Verification items for the finished model (mm, model axes). Face numbers are marked on the shaded views. A direction names the side the tool comes from. Give positions to 0.01 mm unless a question says otherwise; leave off trailing zeros. Answer as a JSON object with one key per item and string values. Group by question number.
(1) Mould release check, pull along Y, two halves, no side actions. Record for the marked faces 1 and 2: +Y half, -Y half, draft (parallel to the pull), parting line (faces both ways), or undercut.
(2) Section check A-A (z = 7.25). Count the separate pieces of the cut face and the enclosed holes in it, then the cut area to 3 significant figures.
(3) Thickness scan on line 1 (Y direction, x = 14, z = 4.5); line 2 (Y direction, x = -0.5, z = 9.5); line 3 (Z direction, x = 23, y = 12.5). Record the ranges inside material, lowest first.
(4) Depth check by flat-ended pin: pin 1 Ø0.6 at (x, y) = (21.5, 21) entering from +Z; pin 2 Ø4 at (x, z) = (15.5, 2.5) entering from -Y; pin 3 Ø3 at (x, z) = (-14, 8.5) entering from +Y; pin 4 Ø2 at (y, z) = (2.5, 5.5) entering from -X. Enter the tip coordinate at first touch or a pass-through.
(5) Access from +Z, -Z, +X, -X, +Y, -Y to the whole of each face (thin tool, end or side, straight path). Record for the marked faces 3 and 4.
```python
from build123d import *

# Parameters (mm, degrees)
F0_R     = 30
F1_DEPTH = 3
F3_DEPTH = 10
F5_COUNT = 7
F6_R     = 7
F7_DEPTH = 10
F8_R     = 4
F9_DEPTH = 13.001
F10_R    = 1
F11_R    = 2


with BuildPart() as f1:
    # F0 (on Top) → F1 (new body)
    with BuildSketch(Plane.XY):
        Circle(F0_R)
    extrude(amount=F1_DEPTH)

    # F2 (on face) → F3 (join)
    with BuildSketch(Plane.XY.offset(3)):
        with BuildLine():
            Line((-1.6446796944, 10.4644708335), (0, 10.4520414025))
            add(Edge.make_bspline(
                [(0, 10.4520414025), (-2.2289291518, 13.3403059975), (-6.1904321331, 16.1620932905), (-13.6442423507, 18.8532101818), (-22.3243720829, 17.9140381515), (-24.8817240251, 16.7600659168)],
                knots=[0, 0, 0, 0, 0.3225761243, 0.6326131084, 1, 1, 1, 1], degree=3))
            Line((-24.8817240251, 16.7600659168), (-25.7866161055, 15.3313544682))
            add(Edge.make_bspline(
                [(-1.6446796944, 10.4644708335), (-2.8414923982, 12.2416667658), (-7.1707724103, 15.3826694675), (-14.4971888519, 17.5675164501), (-22.4425556004, 16.8143108506), (-25.7866161055, 15.3313544682)],
                knots=[0, 0, 0, 0, 0.3011184154, 0.6179723344, 1, 1, 1, 1], degree=3))
        make_face()
    extrude(amount=F3_DEPTH)


with BuildPart() as f5_1:
    # F5: instance of F1
    add(f1.part.rotate(Axis((0, 0, 22.8564720601), (0, 0, 1)), 1 * 360 / F5_COUNT))


with BuildPart() as f5_2:
    # F5: instance of F1
    add(f1.part.rotate(Axis((0, 0, 22.8564720601), (0, 0, 1)), 2 * 360 / F5_COUNT))


with BuildPart() as f5_3:
    # F5: instance of F1
    add(f1.part.rotate(Axis((0, 0, 22.8564720601), (0, 0, 1)), 3 * 360 / F5_COUNT))


with BuildPart() as f5_4:
    # F5: instance of F1
    add(f1.part.rotate(Axis((0, 0, 22.8564720601), (0, 0, 1)), 4 * 360 / F5_COUNT))


with BuildPart() as f5_5:
    # F5: instance of F1
    add(f1.part.rotate(Axis((0, 0, 22.8564720601), (0, 0, 1)), 5 * 360 / F5_COUNT))


with BuildPart() as f5_6:
    # F5: instance of F1
    add(f1.part.rotate(Axis((0, 0, 22.8564720601), (0, 0, 1)), 6 * 360 / F5_COUNT))


with BuildPart() as f1_1:
    add(f1.part)

    add(f5_1.part)  # F7 merges F5_1

    add(f5_2.part)  # F7 merges F5_2

    add(f5_3.part)  # F7 merges F5_3

    add(f5_4.part)  # F7 merges F5_4

    add(f5_5.part)  # F7 merges F5_5

    add(f5_6.part)  # F7 merges F5_6
    # F6 (on face) → F7 (join)
    with BuildSketch(Plane.XY.offset(3)):
        Circle(F6_R)
    extrude(amount=F7_DEPTH)

    # F8 (on face) → F9 (cut, through all)
    with BuildSketch(Plane.XY.offset(13)):
        Circle(F8_R)
    extrude(amount=-F9_DEPTH, mode=Mode.SUBTRACT)

    # F10
    f10_edges = [f1_1.edges().sort_by_distance(p)[0] for p in [
        (-18.704694, 23.454944, 0),
    ]]
    fillet(f10_edges, radius=F10_R)

    # F11
    f11_edges = [f1_1.edges().sort_by_distance(p)[0] for p in [
        (-7, 0, 3),
    ]]
    fillet(f11_edges, radius=F11_R)


solid = f1_1.part
```
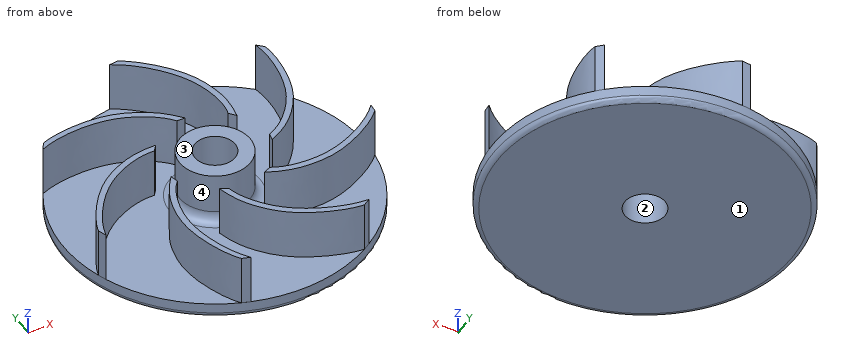
Solutions:
{
 "1": {"face 1": "draft", "face 2": "undercut"},
 "2": {"separate pieces": "8", "enclosed holes": "1", "area": "326 mm2"},
 "3": {"line 1": "y = -25.8 to -24.71, -11.55 to -10.32, -0.09 to 1.47", "line 2": "y = -17.9 to -15.87, -6.98 to -3.97, 3.97 to 6.98, 10.46 to 11.08, 27.23 to 28.66", "line 3": "z = 0 to 3"},
 "4": {"pin 1": "stops at z = 13", "pin 2": "stops at y = -26.79", "pin 3": "stops at y = 18.2", "pin 4": "stops at x = -21.73"},
 "5": {"face 3": "+Z, +X, -X, +Y, -Y", "face 4": "+Z"}
}
